Check sheet for the modelled part. Datum: model origin and axes. Units: mm. A direction names the side the tool comes from. Coordinates: 2 decimals unless noted, no trailing zeros. Loops run counter-clockwise (first coordinate to the right, second up) from the corner with the lowest first, then second, coordinate; pieces in that order, holes last. Notation, with made-up numbers: (56.5, 49) - (86.5, 49) arc R23 ccw to (86.5, 68) - close; hole circle Ø7 at (56, 10.5). An arc over 180 degrees is marked (long way). Use a Markdown table: item, result. Add a question column.
1) Go/stop test with flat-tipped pins: P1, Ø8, axis at x = 3.5, y = 74.5, coming from the -Z side; P2, Ø3, axis at y = 124.5, z = -4.5, coming from the -X side; P3, Ø6, axis at y = 75.5, z = 10, coming from the +X side. Record where each tip stops, or that it passes through.
2) Thickness scan on line 1 (Y direction, x = 14, z = 21); line 2 (Y direction, x = -8.5, z = -14.5); line 3 (Y direction, x = -2, z = 8.5). Record the ranges inside material, lowest first.
3) Tool access check on faces 1 (the cylindrical face through (5.506, 176.494, 24.796)), 2 (the flat face through (-22.5, 173.99, -9.3)). Record the directions out of +Z, -Z, +X, -X, +Y, -Y that give a thin tool (end or side, any length) a straight path to the whole face; none if there is none.
4) Sectioned sample at C-C, the plane y = 49. Enter the section's corners in (x, z).
5) Sectioned sample at D-D, the plane y = 243. Enter the section's corners in (x, z).
Autodesk Inventor part; units mm, degrees
ref_plane "YZ Plane" through (0, 0, 0) normal (1, 0, 0) x (0, 1, 0)
ref_plane "XZ Plane" through (0, 0, 0) normal (0, 1, 0) x (-1, 0, 0)
ref_plane "XY Plane" through (0, 0, 0) normal (0, 0, 1) x (1, 0, 0)
sketch "Sketch1" plane through (0, 0, 0) normal (0, 1, 0) x (-1, 0, 0)
  line L0 (0, -35.56) -> (0, 35.56)
  line L1 (-35.56, 0) -> (35.56, 0)
  circle A0 centre (0, 0) radius 25.4
  dimension "d0" = 50.8
extrude "Extrusion1" add sketch "Sketch1" along normal blind 279.4
sketch "Sketch2" plane through (0, 0, 0) normal (1, 0, 0) x (0, 1, 0)
  line L0 (279.4, -25.4) -> (279.4, 25.4)
  line L1 (0, 25.4) -> (0, -25.4)
  line L2 (0, -25.4) -> (279.4, -25.4)
  line L3 (0, 25.4) -> (10.16, 25.4)
  line L4 (10.16, 25.4) -> (10.16, -25.4)
  line L5 (10.16, -25.4) -> (0, -25.4)
  line L6 (0, -25.4) -> (0, 25.4)
  line L7 (-5.08, 12.7) -> (25.4, 12.7)
  line L8 (25.4, 12.7) -> (25.4, -12.7)
  line L9 (25.4, -12.7) -> (-5.08, -12.7)
  line L10 (-5.08, -12.7) -> (-5.08, 12.7)
  line L11 (-5.08, 12.7) -> (25.4, -12.7) construction
  line L12 (25.4, 12.7) -> (-5.08, -12.7) construction
  line L13 (-27.94, 8.6578) -> (78.74, 8.6578)
  line L14 (78.74, 8.6578) -> (78.74, -8.6578)
  line L15 (78.74, -8.6578) -> (-27.94, -8.6578)
  line L16 (-27.94, -8.6578) -> (-27.94, 8.6578)
  line L17 (-27.94, 8.6578) -> (78.74, -8.6578) construction
  line L18 (78.74, 8.6578) -> (-27.94, -8.6578) construction
  line L19 (78.74, 25.4) -> (0, 25.4)
  line L20 (0, 25.4) -> (0, -25.4)
  line L21 (0, -25.4) -> (78.74, -25.4)
  line L22 (78.74, -25.4) -> (78.74, 25.4)
  line L23 (25.4, 8.6578) -> (78.74, 8.6578)
  line L24 (78.74, 8.6578) -> (78.74, 25.4)
  line L25 (78.74, 25.4) -> (25.4, 25.4)
  line L26 (25.4, 25.4) -> (25.4, 8.6578)
  line L27 (10.16, 12.7) -> (25.4, 12.7)
  line L28 (25.4, 12.7) -> (25.4, 25.4)
  line L29 (25.4, 25.4) -> (10.16, 25.4)
  line L30 (10.16, 25.4) -> (10.16, 12.7)
  line L31 (10.16, -12.7) -> (25.4, -12.7)
  line L32 (25.4, -12.7) -> (25.4, -25.4)
  line L33 (25.4, -25.4) -> (10.16, -25.4)
  line L34 (10.16, -25.4) -> (10.16, -12.7)
  line L35 (25.4, -8.6578) -> (78.74, -8.6578)
  line L36 (78.74, -8.6578) -> (78.74, -25.4)
  line L37 (78.74, -25.4) -> (25.4, -25.4)
  line L38 (25.4, -25.4) -> (25.4, -8.6578)
  line L39 (-89.408, 0) -> (340.868, 0)
  point P0 (0, 0)
  point P1 (10.16, 0)
  point P2 (25.4, 0)
  dimension "d3" = 10.16
  dimension "d4" = 30.48
  dimension "d5" = 25.4
  dimension "d6" = 106.68
revolve "Revolution1" cut sketch "Sketch2" angle 360 about axis through (0, -10, 0) along (0, 1, 0) contours L2 L32 L8 L15 L22 | L2 L4 L9 L32 | L13 L8 L26 L19 L22 | L7 L4 L19 L26
sketch "Sketch3" plane through (0, 0, 0) normal (0, 0, 1) x (1, 0, 0)
  line L0 (25.4, 78.74) -> (-25.4, 78.74)
  line L1 (25.4, 78.74) -> (-25.4, 78.74)
  line L2 (25.4, 279.4) -> (-25.4, 279.4)
  line L3 (-25.4, 78.74) -> (25.4, 78.74)
  line L4 (25.4, 78.74) -> (25.4, 279.4)
  line L5 (25.4, 279.4) -> (-25.4, 279.4)
  line L6 (-25.4, 279.4) -> (-25.4, 78.74)
  line L7 (-25.4, 78.74) -> (-25.4, 279.4)
  line L8 (25.4, 279.4) -> (-25.4, 279.4)
  line L9 (-25.4, 279.4) -> (-25.4, 269.24)
  line L10 (-25.4, 269.24) -> (25.4, 269.24)
  line L11 (25.4, 269.24) -> (25.4, 279.4)
  line L12 (25.4, 78.74) -> (25.4, 279.4)
  line L13 (-25.4, 269.24) -> (25.4, 269.24)
  line L14 (25.4, 269.24) -> (25.4, 228.6)
  line L15 (25.4, 228.6) -> (-25.4, 228.6)
  line L16 (-25.4, 228.6) -> (-25.4, 269.24)
  line L17 (25.4, 228.6) -> (-25.4, 228.6)
  line L18 (-25.4, 228.6) -> (-25.4, 223.52)
  line L19 (-25.4, 223.52) -> (25.4, 223.52)
  line L20 (25.4, 223.52) -> (25.4, 228.6)
  line L21 (-25.4, 223.52) -> (15.24, 223.52)
  line L22 (15.24, 223.52) -> (15.24, 179.07)
  line L23 (15.24, 179.07) -> (-25.4, 179.07)
  line L24 (-25.4, 179.07) -> (-25.4, 223.52)
  line L25 (25.4, 179.07) -> (-25.4, 179.07)
  line L26 (-25.4, 179.07) -> (-25.4, 173.99)
  line L27 (-25.4, 173.99) -> (25.4, 173.99)
  line L28 (25.4, 173.99) -> (25.4, 179.07)
  line L29 (-25.4, 173.99) -> (25.4, 173.99)
  line L30 (25.4, 173.99) -> (25.4, 133.35)
  line L31 (25.4, 133.35) -> (-25.4, 133.35)
  line L32 (-25.4, 133.35) -> (-25.4, 173.99)
  line L33 (0, 269.24) -> (-24.13, 269.24)
  line L34 (-24.13, 269.24) -> (-24.13, 228.6)
  line L35 (-24.13, 228.6) -> (0, 228.6)
  line L36 (0, 228.6) -> (0, 269.24)
  line L37 (-25.4, 228.6) -> (-24.13, 228.6)
  line L38 (-24.13, 228.6) -> (-24.13, 269.24)
  line L39 (-24.13, 269.24) -> (-25.4, 269.24)
  line L40 (-25.4, 269.24) -> (-25.4, 228.6)
  line L41 (-25.4, 179.07) -> (-24.13, 179.07)
  line L42 (-24.13, 179.07) -> (-24.13, 223.52)
  line L43 (-24.13, 223.52) -> (-25.4, 223.52)
  line L44 (-25.4, 223.52) -> (-25.4, 179.07)
  line L45 (-25.4, 173.99) -> (-24.13, 173.99)
  line L46 (-24.13, 173.99) -> (-24.13, 133.35)
  line L47 (-24.13, 133.35) -> (-25.4, 133.35)
  line L48 (-25.4, 133.35) -> (-25.4, 173.99)
  point P0 (0, 0)
  dimension "d8" = 10.16
  dimension "d9" = 40.64
  dimension "d10" = 5.08
  dimension "d11" = 40.64
  dimension "d12" = 5.08
  dimension "d13" = 40.64
  dimension "d14" = 24.13
  dimension "d15" = 1.27
  dimension "d16" = 1.27
  dimension "d17" = 40.64
revolve "Revolution2" cut sketch "Sketch3" angle 360 about axis through (0, 228.6, 0) along (0, 1, 0) contours L6 L27 L46 L31 | L6 L19 L42 L23 | L6 L10 L34 L15
properties part number "TowerLight" material "UHMW, White"
Solved:
| question | item | result |
|---|---|---|
| 1 | P1 | stops at z = -8.66 |
| 1 | P2 | stops at x = -25.22 |
| 1 | P3 | stops at x = 5.09 |
| 2 | line 1 | y = 0 to 10.16, 78.74 to 133.35, 173.99 to 179.07, 223.52 to 228.6, 269.24 to 279.4 |
| 2 | line 2 | y = 0 to 10.16, 78.74 to 279.4 |
| 2 | line 3 | y = 0 to 25.4, 78.74 to 279.4 |
| 3 | face 1 | +Y, -Y |
| 3 | face 2 | none |
| 4 | outline | circle Ø17.32 at (0, 0) |
| 5 | outline | circle Ø48.26 at (0, 0) |
